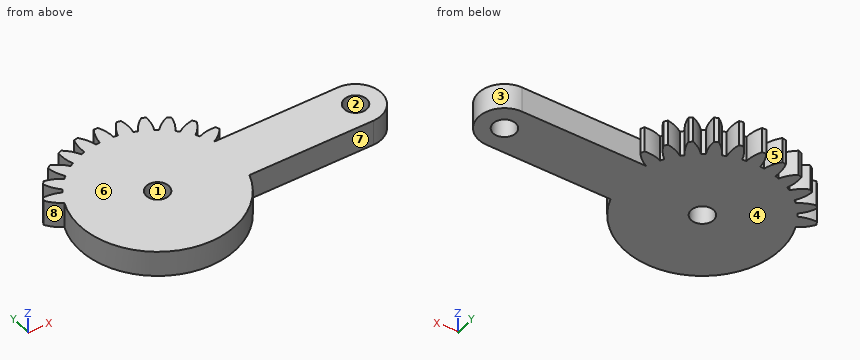
```python
from build123d import *

# Parameters (mm, degrees)
SKETCH1_R           = 1.75
BOSS_EXTRUDE2_DEPTH = 4


with BuildPart() as part:
    # Sketch1 → Boss-Extrude2 (new body)
    # profile 1 of 12: a face of its own
    with BuildSketch(Plane.XY):
        with BuildLine():
            Line((30.5, -4), (11.419719786, -4))
            ThreePointArc((11.419719786, -4), (-12.1, 0), (11.419719786, 4))
            Line((11.419719786, 4), (30.5, 4))
            ThreePointArc((30.5, 4), (34.5, 0), (30.5, -4))
        make_face()
        Circle(SKETCH1_R, mode=Mode.SUBTRACT)
        with Locations((30.5, 0)):
            Circle(SKETCH1_R, mode=Mode.SUBTRACT)
    # profile 2 of 12: a face of its own
    with BuildSketch(Plane.XY):
        with BuildLine():
            ThreePointArc((2.04630572, 11.925713098), (3.062574606, 11.706008576), (4.056229837, 11.399868399))
            ThreePointArc((4.056229837, 11.399868399), (4.191789848, 12.739862338), (4.004557713, 14.073618088))
            Line((4.004557713, 14.073618088), (3.400741544, 14.231598069))
            ThreePointArc((3.400741544, 14.231598069), (2.585583316, 13.159679272), (2.04630572, 11.925713098))
        make_face()
    # profile 3 of 12: a face of its own
    with BuildSketch(Plane.XY):
        with BuildLine():
            ThreePointArc((-0.641917286, 12.082960821), (0.397776079, 12.093459976), (1.434532317, 12.014662585))
            ThreePointArc((1.434532317, 12.014662585), (1.27037575, 13.351454601), (0.792800193, 14.610772615))
            Line((0.792800193, 14.610772615), (0.168997044, 14.631297504))
            ThreePointArc((0.168997044, 14.631297504), (-0.388904138, 13.405638858), (-0.641917286, 12.082960821))
        make_face()
    # profile 4 of 12: a face of its own
    with BuildSketch(Plane.XY):
        with BuildLine():
            ThreePointArc((-3.071117398, 14.306350498), (-3.344130279, 12.987655382), (-3.298347959, 11.641773952))
            ThreePointArc((-3.298347959, 11.641773952), (-2.286723162, 11.881956791), (-1.258213497, 12.034404796))
            ThreePointArc((-1.258213497, 12.034404796), (-1.713956435, 13.301787393), (-2.458222459, 14.424297241))
            Line((-2.458222459, 14.424297241), (-3.071117398, 14.306350498))
        make_face()
    # profile 5 of 12: a face of its own
    with BuildSketch(Plane.XY):
        with BuildLine():
            ThreePointArc((-6.159128153, 13.272850751), (-6.133731183, 11.926430371), (-5.791420864, 10.624003218))
            ThreePointArc((-5.791420864, 10.624003218), (-4.857967527, 11.08197417), (-3.888643585, 11.458117257))
            ThreePointArc((-3.888643585, 11.458117257), (-4.613401246, 12.593320589), (-5.587496363, 13.523427559))
            Line((-5.587496363, 13.523427559), (-6.159128153, 13.272850751))
        make_face()
    # profile 6 of 12: a face of its own
    with BuildSketch(Plane.XY):
        with BuildLine():
            ThreePointArc((-8.942094855, 11.581984556), (-8.619545875, 10.274523276), (-7.997661209, 9.080055902))
            ThreePointArc((-7.997661209, 9.080055902), (-7.188610613, 9.733132972), (-6.326480245, 10.314341845))
            ThreePointArc((-6.326480245, 10.314341845), (-7.28435745, 11.261142529), (-8.440037507, 11.952781076))
            Line((-8.440037507, 11.952781076), (-8.942094855, 11.581984556))
        make_face()
    # profile 7 of 12: a face of its own
    with BuildSketch(Plane.XY):
        with BuildLine():
            ThreePointArc((-11.2821851, 9.317495695), (-10.67845904, 8.113748343), (-9.807800202, 7.086399311))
            ThreePointArc((-9.807800202, 7.086399311), (-9.163222316, 7.902237454), (-8.450984381, 8.659726496))
            ThreePointArc((-8.450984381, 8.659726496), (-9.594540202, 9.371232193), (-10.874567661, 9.790147432))
            Line((-10.874567661, 9.790147432), (-11.2821851, 9.317495695))
        make_face()
    # profile 8 of 12: a face of its own
    with BuildSketch(Plane.XY):
        with BuildLine():
            ThreePointArc((-13.06350089, 6.591537844), (-12.208498581, 5.551122593), (-11.13218682, 4.741773571))
            ThreePointArc((-11.13218682, 4.741773571), (-10.684005749, 5.67996665), (-10.15693536, 6.576219589))
            ThreePointArc((-10.15693536, 6.576219589), (-11.42953274, 7.017191451), (-12.770511491, 7.142635705))
            Line((-12.770511491, 7.142635705), (-13.06350089, 6.591537844))
        make_face()
    # profile 9 of 12: a face of its own
    with BuildSketch(Plane.XY):
        with BuildLine():
            ThreePointArc((4.633181039, 11.177818815), (5.575692546, 10.738791954), (6.47703386, 10.22047124))
            ThreePointArc((6.47703386, 10.22047124), (6.905596548, 11.497301024), (7.017980909, 12.839437391))
            Line((7.017980909, 12.839437391), (6.464057014, 13.127048167))
            ThreePointArc((6.464057014, 13.127048167), (5.432014202, 12.2619583), (4.633181039, 11.177818815))
        make_face()
    # profile 10 of 12: a face of its own
    with BuildSketch(Plane.XY):
        with BuildLine():
            ThreePointArc((6.990588114, 9.876319042), (7.812662335, 9.239713591), (8.577048867, 8.534883288))
            ThreePointArc((8.577048867, 8.534883288), (9.277388744, 9.685311177), (9.683823524, 10.969355975))
            Line((9.683823524, 10.969355975), (9.207226173, 11.372353004))
            ThreePointArc((9.207226173, 11.372353004), (8.009412915, 10.7569375), (6.990588114, 9.876319042))
        make_face()
    # profile 11 of 12: a face of its own
    with BuildSketch(Plane.XY):
        with BuildLine():
            ThreePointArc((9.001771295, 8.085673352), (9.662693238, 7.283018563), (10.252267103, 6.426586905))
            ThreePointArc((10.252267103, 6.426586905), (11.189698333, 7.393635488), (11.870053976, 8.555993639))
            Line((11.870053976, 8.555993639), (11.494387677, 9.054417628))
            ThreePointArc((11.494387677, 9.054417628), (10.190128247, 8.719156263), (9.001771295, 8.085673352))
        make_face()
    # profile 12 of 12: a face of its own
    with BuildSketch(Plane.XY):
        with BuildLine():
            ThreePointArc((10.567122415, 5.894567319), (11.034158501, 4.965616394), (11.419719786, 4))
            ThreePointArc((11.419719786, 4), (12.547814073, 4.735774119), (13.468394505, 5.718877338))
            Line((13.468394505, 5.718877338), (13.212264939, 6.288042768))
            ThreePointArc((13.212264939, 6.288042768), (11.866155587, 6.249540081), (10.567122415, 5.894567319))
        make_face()
    extrude(amount=BOSS_EXTRUDE2_DEPTH)


solid = part.part
```
Part model, mm, in its own coordinate system. Face numbers are marked on the shaded views. A direction names the side the tool comes from. Coordinates: 2 decimals unless noted, no trailing zeros. Write each loop counter-clockwise with the first axis right and the second up, starting at its lowest first coordinate (ties: lowest second). Pieces come first, ordered by that corner, then holes.
Item 1: Slice it at D-D (y = -7.75). Write the cut outline in (x, z).
Item 2: Probe line 1 (Y direction, x = 30.5, z = 1.8); line 2 (X direction, y = 10.75, z = 0.4); line 3 (X direction, y = 1.5, z = 1.7). List the from-to ranges inside material, lowest first.
Item 3: Slice it at C-C (z = 1.15). Count the separate pieces of the cut face and the enclosed holes in it, and give its area (3 significant figures).
Item 4: Mould opens along X. For the marked faces 1, 2, 3 and 4 say: released by +X, released by -X, zero draft, split by the parting line, or undercut.
Item 5: Pin check, flat tip, straight feed: pin 1 (1.5 mm diameter, centred on y = 0, z = 3.5, fed in from -X). Stop position of the tip, or through.
Item 6: Slice it at B-B (x = 25). Write the cut outline in (y, z), and give its area (3 significant figures).
Item 7: Slice it at A-A (y = 0). Write the cut outline in (x, z), and give its area (3 significant figures).
Item 8: Which spindle directions (+Z, -Z, +X, -X, +Y, -Y) get a long thin tool onto all of the face, cutting with end or side? Do the marked faces 5, 6, 7 and 8. Say none if no direction does.
Results found:
1. outline: (-9.29, 0) - (9.29, 0) - (9.29, 4) - (-9.29, 4) - close
2. line 1: y = -4 to -1.75, 1.75 to 4
2. line 2: x = -8.78 to -6.71, -5.84 to 6.7, 8 to 9.64
2. line 3: x = -12.01 to -0.9, 0.9 to 29.6, 31.4 to 34.21
3. separate pieces: 1
3. enclosed holes: 2
3. area: 659 mm2
4. face 1: undercut
4. face 2: undercut
4. face 3: released by +X
4. face 4: zero draft
5. pin 1: stops at x = -12.1
6. outline: (-4, 0) - (4, 0) - (4, 4) - (-4, 4) - close
6. area: 32.0 mm2
7. outline: (-12.1, 0) - (-1.75, 0) - (-1.75, 4) - (-12.1, 4) - close; (1.75, 0) - (28.75, 0) - (28.75, 4) - (1.75, 4) - close; (32.25, 0) - (34.5, 0) - (34.5, 4) - (32.25, 4) - close
7. area: 158 mm2
8. face 5: +Z, -Z, +Y
8. face 6: +Z, +X, -X, +Y, -Y
8. face 7: +Z, -Z, +X, -Y
8. face 8: +Z, -Z, -X
